```python
from build123d import *

# Parameters (mm, degrees)
SKETCH1_R           = 7.5
BOSS_EXTRUDE1_DEPTH = 5
SKETCH2_R           = 8.5
BOSS_EXTRUDE2_DEPTH = 2
SKETCH3_R           = 7.5
BOSS_EXTRUDE3_DEPTH = 35
SKETCH4_R           = 4
CUT_EXTRUDE1_DEPTH  = 20.5
SKETCH6_W           = 3
SKETCH6_H           = 1.5
CUT_EXTRUDE2_DEPTH  = 20.5
CUT_EXTRUDE3_REACH  = 47.741
SKETCH7_R           = 1
CUT_EXTRUDE5_START  = -35
SKETCH8_W           = 5
SKETCH8_H           = 4
CUT_EXTRUDE5_DEPTH  = 19
CUT_EXTRUDE6_START  = -14
SKETCH9_R           = 7.5
SKETCH9_R_2         = 7
CUT_EXTRUDE6_DEPTH  = 14
FILLET1_R           = 0.8


with BuildPart() as part:
    # Sketch1 → Boss-Extrude1 (new body)
    with BuildSketch(Plane(origin=(0, 0, 0), x_dir=(0, 0, -1), z_dir=(1, 0, 0))):
        Circle(SKETCH1_R)
    extrude(amount=BOSS_EXTRUDE1_DEPTH)

    # Sketch2 → Boss-Extrude2 (add)
    with BuildSketch(Plane(origin=(5, 0, 0), x_dir=(0, 0, -1), z_dir=(1, 0, 0))):
        Circle(SKETCH2_R)
    extrude(amount=BOSS_EXTRUDE2_DEPTH)

    # Sketch3 → Boss-Extrude3 (add)
    with BuildSketch(Plane(origin=(7, 0, 0), x_dir=(0, 0, -1), z_dir=(1, 0, 0))):
        Circle(SKETCH3_R)
    extrude(amount=BOSS_EXTRUDE3_DEPTH)

    # Sketch4 → Cut-Extrude1 (cut)
    with BuildSketch(Plane.ZY):
        Circle(SKETCH4_R)
    extrude(amount=-CUT_EXTRUDE1_DEPTH, mode=Mode.SUBTRACT)

    # Sketch6 → Cut-Extrude2 (cut)
    with BuildSketch(Plane.ZY):
        with Locations((0, 4)):
            Rectangle(SKETCH6_W, SKETCH6_H)
    extrude(amount=-CUT_EXTRUDE2_DEPTH, mode=Mode.SUBTRACT)

    # Sketch7 → Cut-Extrude3 (cut, up to next)
    with BuildSketch(Plane(origin=(0, 7.5, 0), x_dir=(1, 0, 0), z_dir=(0, 1, 0)), mode=Mode.PRIVATE) as cut_extrude3_sk1:
        with Locations(Location((12, 0, 0), (0, 0, 270))):
            Circle(SKETCH7_R)
    cut_extrude3_tool1 = extrude(cut_extrude3_sk1.sketch, amount=-CUT_EXTRUDE3_REACH, mode=Mode.PRIVATE) & part.part
    add(cut_extrude3_tool1.solids().sort_by_distance((12, 7.5, 0))[0], mode=Mode.SUBTRACT)

    # Sketch8 → Cut-Extrude5 (cut)
    with BuildSketch(Plane(origin=(42, 0, 0), x_dir=(0, 0, -1), z_dir=(1, 0, 0)).offset(CUT_EXTRUDE5_START)):
        with Locations((0, -7.5)):
            Rectangle(SKETCH8_W, SKETCH8_H)
    extrude(amount=CUT_EXTRUDE5_DEPTH, mode=Mode.SUBTRACT)

    # Sketch9 → Cut-Extrude6 (cut)
    with BuildSketch(Plane(origin=(42, 0, 0), x_dir=(0, 0, -1), z_dir=(1, 0, 0)).offset(CUT_EXTRUDE6_START)):
        with Locations(Location((0, 0, 0), (0, 0, 250.528779366))):
            Circle(SKETCH9_R)
        Circle(SKETCH9_R_2, mode=Mode.SUBTRACT)
    extrude(amount=CUT_EXTRUDE6_DEPTH, mode=Mode.SUBTRACT)

    # Fillet1
    # the kernel refuses this fillet: 0.8 mm, written as the material it adds along each edge
    with BuildSketch(Plane(origin=(28, 0, 0), x_dir=(0, 0, -1), z_dir=(0, -1, 0))) as fillet1_piece_1:
        with BuildLine():
            CenterArc((7.8, 0.741619849), FILLET1_R, 180, 67.975687163)
            Line((7, 0.741619849), (6.984, 0.741619849))
            Line((6.984, 0.741619849), (6.984, 0))
            Line((6.984, 0), (7, -0.016))
            ThreePointArc((7, -0.016), (7.25, -0.016), (7.494, -0.014832397))
            Line((7.494, -0.014832397), (7.5, 0))
        make_face()
    revolve(axis=Axis((28, 0, 0), (1, 0, 0)))


solid = part.part
```
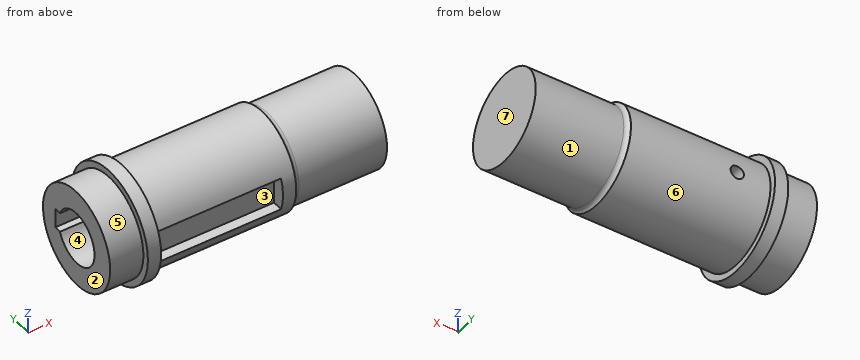
Build history of the part. All positions in model axes, mm. Face numbers are marked on the shaded views. A direction names the side the tool comes from. Round coordinates to 2 decimals unless told otherwise and drop trailing zeros. Write each loop counter-clockwise with the first axis right and the second up, starting at its lowest first coordinate (ties: lowest second). Pieces come first, ordered by that corner, then holes.
1) Band-saw the part on D-D, the plane x = 6.5. List the corners of the cut face in (y, z).
2) Band-saw the part on A-A, the plane z = 0. List the corners of the cut face in (x, y), and give its area (3 significant figures).
3) Pin check, flat tips, straight feed: pin 1 (0.8 mm diameter, centred on x = 6, y = 4, fed in from -Z); pin 2 (8 mm diameter, centred on x = 25, y = -3, fed in from -Z); pin 3 (2 mm diameter, centred on x = 30, y = -0.5, fed in from -Z). Stop position of each tip, or through.
4) Band-saw the part on C-C, the plane y = 0. List the corners of the cut face in (x, z), and give its area (3 significant figures).
5) Band-saw the part on B-B, the plane x = 16. List the corners of the cut face in (y, z).
6) Drill centre lines: probe 1 along Z at (x, y) = (15.5, 0); probe 2 along X at (y, z) = (5.8, 0); probe 3 along Y at (x, z) = (13.75, 0). Where is each one in solid material? Low to high.
7) Mould opens along Y. For the marked faces 1, 2, 3 and 4 say: +Y half, -Y half, draft (parallel to the pull), parting line (faces both ways), or undercut.
8) 3-axis set-ups, long thin cutter, end or side, ignore diameter. For the marked faces 5, 6 and 7: which of +Z, -Z, +X, -X, +Y, -Y reach the whole face in a straight line?
Ans:
1. outline: circle Ø17 at (0, 0); hole (3.71, -1.5) - (4.75, -1.5) - (4.75, 1.5) - (3.71, 1.5) arc R4 ccw (long way) to start
2. outline: (0, -7.5) - (5, -7.5) - (5, -8.5) - (7, -8.5) - (7, -5.5) - (26, -5.5) - (26, -7.5) - (28, -7.5) arc R0.8 cw to (28.74, -7) - (42, -7) - (42, 7) - (28.74, 7) arc R0.8 cw to (28, 7.5) - (13, 7.5) - (13, 4.75) - (20.5, 4.75) - (20.5, -4) - (0, -4) - close; (0, 4.75) - (11, 4.75) - (11, 7.5) - (7, 7.5) - (7, 8.5) - (5, 8.5) - (5, 7.5) - (0, 7.5) - close
2. area: 397 mm2
3. pin 1: stops at z = -7.7
3. pin 2: stops at z = -7.5
3. pin 3: stops at z = -7
4. outline: (0, -7.5) - (5, -7.5) - (5, -8.5) - (7, -8.5) - (7, -7.5) - (28, -7.5) arc R0.8 cw to (28.74, -7) - (42, -7) - (42, 7) - (28.74, 7) arc R0.8 cw to (28, 7.5) - (7, 7.5) - (7, 8.5) - (5, 8.5) - (5, 7.5) - (0, 7.5) - (0, 4) - (20.5, 4) - (20.5, -4) - (0, -4) - close
4. area: 456 mm2
5. outline: (-7.07, -2.5) arc R7.5 ccw (long way) to (-7.07, 2.5) - (-5.5, 2.5) - (-5.5, -2.5) - close; hole (3.71, -1.5) - (4.75, -1.5) - (4.75, 1.5) - (3.71, 1.5) arc R4 ccw (long way) to start
6. probe 1: z = -7.5 to -4, 4 to 7.5
6. probe 2: x = 0 to 11, 13 to 42
6. probe 3: y = -5.5 to -4, 4.75 to 7.5
7. face 1: parting line
7. face 2: draft
7. face 3: -Y half
7. face 4: undercut
8. face 5: -X
8. face 6: +X
8. face 7: +Z, -Z, +X, +Y, -Y
